Input: dimensioned drawing with shaded views. Units: mm. Origin: part minimum x, y, z. A direction names the side the tool comes from. Give positions to 0.01 mm unless a question says otherwise; leave off trailing zeros. Loops run counter-clockwise (first coordinate to the right, second up) from the corner with the lowest first, then second, coordinate; pieces in that order, holes last. Notation, with made-up numbers: (-11, 48.5) -> (-3, 48.5) arc R10 ccw to (-3, 62.5) -> close; hole circle Ø1 at (15.25, 26.5). An arc over 180 degrees is marked (long way). Answer in a Markdown table with one row per item. Add a question column.
1) First-contact query: P1, Ø7.5, axis at x = 52, z = 34, coming from the -Y side; P2, Ø5, axis at y = 17, z = 38, coming from the +X side; P3, Ø11.5, axis at x = 57.5, y = 9.5, coming from the -Z side (3 decimals); P4, Ø2, axis at y = 13, z = 15, coming from the -X side. Flat tips, straight axial feed; report the tip coordinate or a pass-through.
2) Section query D-D (z = 30). Return the cut outline in (x, y), plus the area to 3 significant figures.
3) Access query for the marked faces 1, 2, 3 and 4. Directions: +Z, -Z, +X, -X, +Y, -Y. A direction counts if a zero-diameter tool reaches every point of the face in a straight line with its end or side. Return the directions, or none.
4) Line query: line 1 (X direction, y = 3, z = 38); line 2 (X direction, y = 9, z = 38); line 3 (Z direction, x = 26, y = 16). Output: solid intervals per line, ascending. Write a range as from..to.
5) Draft query along X for the marked faces 5, 6 and 7. Return one class per face: +X half, -X half, draft (parallel to the pull), parting line (faces both ways), or undercut.
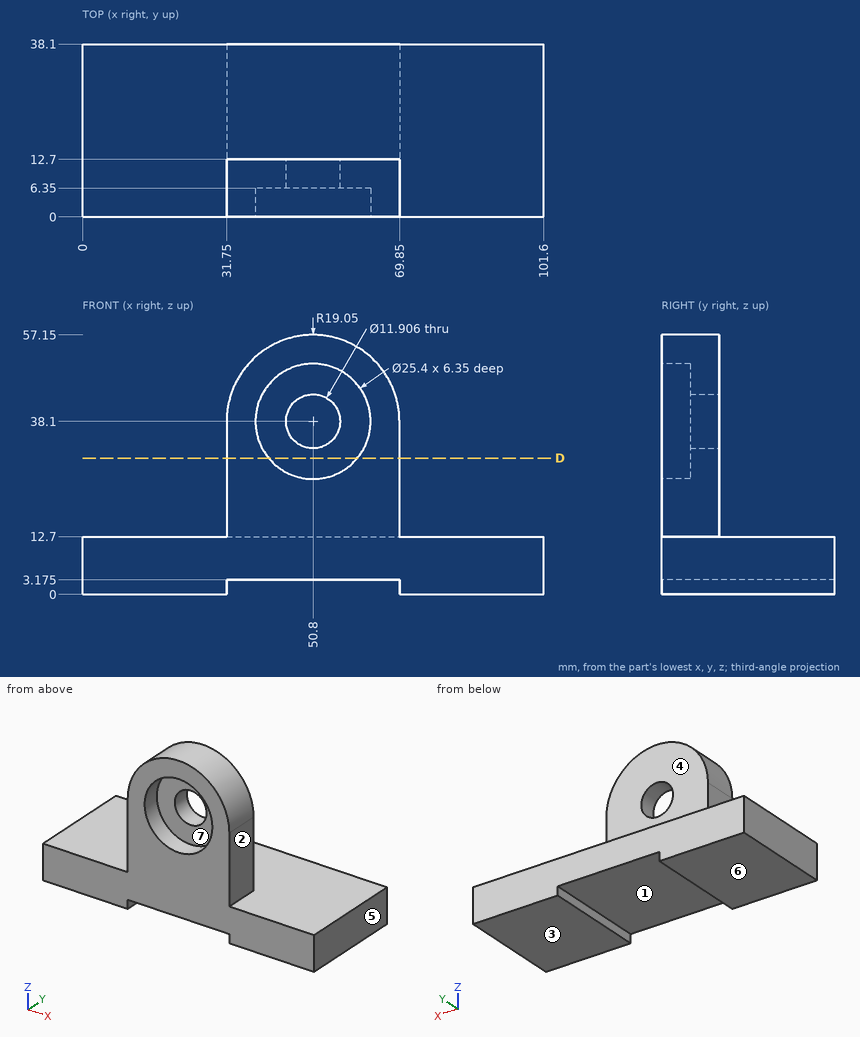
Evaluation:
| question | item | result |
|---|---|---|
| 1 | P1 | y = 6.35 |
| 1 | P2 | through |
| 1 | P3 | z = 3.175 |
| 1 | P4 | x = 31.75 |
| 2 | outline | (31.75, 0) -> (41.02, 0) -> (41.02, 6.35) -> (60.58, 6.35) -> (60.58, 0) -> (69.85, 0) -> (69.85, 12.7) -> (31.75, 12.7) -> close |
| 2 | area | 360 mm² |
| 3 | face 1 | -Z, +Y, -Y |
| 3 | face 2 | +Z, +X, +Y, -Y |
| 3 | face 3 | -Z, +X, -X, +Y, -Y |
| 3 | face 4 | +Z, +X, -X, +Y |
| 4 | line 1 | 31.75..38.1, 63.5..69.85 |
| 4 | line 2 | 31.75..44.85, 56.75..69.85 |
| 4 | line 3 | 0..12.7 |
| 5 | face 5 | +X half |
| 5 | face 6 | draft |
| 5 | face 7 | undercut |
